The drawing under review shows one solid part. Ordinate dimensions are in mm from its lowest x, y, z. A direction names the side the tool comes from. Coordinates: 2 decimals unless noted, no trailing zeros. Write each loop counter-clockwise with the first axis right and the second up, starting at its lowest first coordinate (ties: lowest second). Pieces come first, ordered by that corner, then holes. Notation, with made-up numbers: (55, -25.75) - (94, -25.75) arc R6 ccw to (94, -15.75) - close; hole circle Ø2 at (31, 38.5). An arc over 180 degrees is marked (long way). Put each result on its own line as item: value. Start each with the question number.
Item 1: For pin 1 (3 mm diameter, centred on x = 4, z = 10.5, fed in from +Y); pin 2 (1.5 mm diameter, centred on x = 31.5, z = 2, fed in from -Y); pin 3 (3 mm diameter, centred on y = 6.5, z = 7, fed in from +X), all flat-tipped, find the tip position at first contact; note any pin that passes through.
Item 2: Consider section B-B on z = 6.25. Give the boundary of the cut face in (x, y).
Item 3: Consider section D-D on x = 35. Give the boundary of the cut face in (y, z).
Item 4: Mouldability with a two-part tool opening along Z and no side actions: class the marked faces 4, 5 and 6 as pulls with the +Z half, pulls with the -Z half, needs draft (parallel to the pull), parting line crosses it, or undercut.
Item 5: To check wall thickness, follow L1, parallel to X at y = 2.75, z = 5; L2, parallel to X at y = 5, z = 7.5; L3, parallel to Y at x = 32.5, z = 1.75. State the ranges of each line that lie inside material, in increasing order. Write a range as [from, to].
Item 6: Consider section A-A on y = 13.75. Give the boundary of the cut face in (x, z).
Item 7: Machinability: for the marked faces 1, 2 and 3, which of the approach directions +Z, -Z, +X, -X, +Y, -Y give a long, thin tool a straight path to every point of the face, cutting with its end or side? Answer none if there is none.
Item 8: Consider section C-C on y = 7. Give the boundary of the cut face in (x, z).
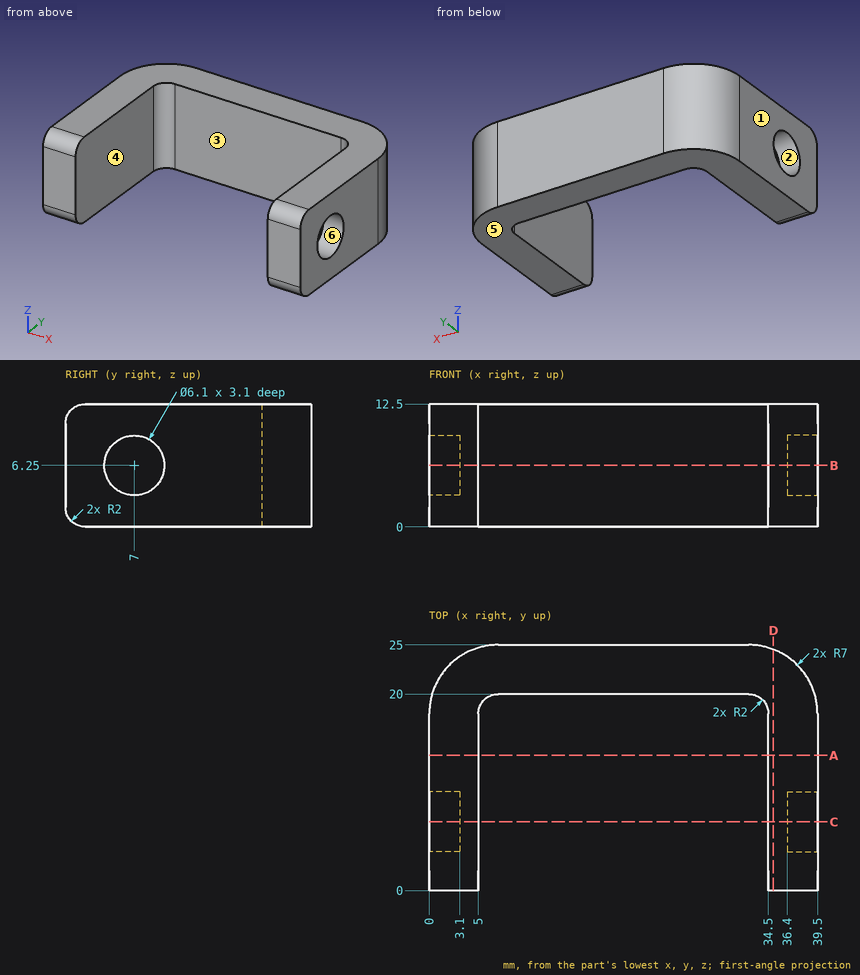
Report:
1. pin 1: y = 24.84
1. pin 2: y = 20
1. pin 3: x = 36.4
2. outline: (0, 0) - (5, 0) - (5, 18) arc R2 cw to (7, 20) - (32.5, 20) arc R2 cw to (34.5, 18) - (34.5, 0) - (39.5, 0) - (39.5, 3.95) - (36.4, 3.95) - (36.4, 10.05) - (39.5, 10.05) - (39.5, 18) arc R7 ccw to (32.5, 25) - (7, 25) arc R7 ccw to (0, 18) - (0, 10.05) - (3.1, 10.05) - (3.1, 3.95) - (0, 3.95) - close
3. outline: (0, 2) arc R2 ccw to (2, 0) - (24.54, 0) - (24.54, 12.5) - (2, 12.5) arc R2 ccw to (0, 10.5) - close
4. face 4: needs draft
4. face 5: pulls with the -Z half
4. face 6: undercut
5. L1: [0, 5], [34.5, 39.5]
5. L2: [3.1, 5], [34.5, 36.4]
5. L3: [20, 25]
6. outline: (0, 0) - (5, 0) - (5, 12.5) - (0, 12.5) - close; (34.5, 0) - (39.5, 0) - (39.5, 12.5) - (34.5, 12.5) - close
7. face 1: +Z, -Z, -X, +Y, -Y
7. face 2: -X
7. face 3: +Z, -Z, -Y
8. outline: (0, 0) - (5, 0) - (5, 12.5) - (0, 12.5) - (0, 9.3) - (3.1, 9.3) - (3.1, 3.2) - (0, 3.2) - close; (34.5, 0) - (39.5, 0) - (39.5, 3.2) - (36.4, 3.2) - (36.4, 9.3) - (39.5, 9.3) - (39.5, 12.5) - (34.5, 12.5) - close
